Model file for the job. Use its own axes, mm. Face numbers are marked on the shaded views. A direction names the side the tool comes from. Give positions to 0.01 mm unless a question says otherwise; leave off trailing zeros. Loops run counter-clockwise (first coordinate to the right, second up) from the corner with the lowest first, then second, coordinate; pieces in that order, holes last. Notation, with made-up numbers: M -20.5,59 L 4.5,59 A4 ccw 4.5,65 Z; hole C -29.5,-29 d11. An arc over 180 degrees is marked long. Use CSV: the item, a comma, the result in double quotes. Start each with the question number.
(1) Slice it at D-D on x = 5.5. List the corners of the cut face in (y, z), and give its area (3 significant figures).
(2) Slice it at B-B on y = 21.5. List the corners of the cut face in (x, z), and give its area (3 significant figures).
(3) Two-plate mould, pull along Z, no slides. Class the marked faces 6, 7 and 8: pulls with the +Z half, pulls with the -Z half, needs draft (parallel to the pull), parting line crosses it, or undercut.
(4) Tool access for the marked faces 1, 2, 3, 4 and 5: list every direction of +Z, -Z, +X, -X, +Y, -Y with a clear straight run to the whole face (end or side of a thin tool).
(5) Slice it at C-C on z = 0. List the corners of the cut face in (x, y).
(6) Slice it at A-A on x = -3.5. List the corners of the cut face in (y, z).
(7) Flat gauge pins, fed straight in: P1, Ø5, axis at x = -5.5, z = 0, coming from the +Y side; P2, Ø3.5, axis at x = -1, z = 2.5, coming from the +Y side. Where does each tip first touch, or does it go through?
(8) Wall check: line 1 along Z through (x, y) = (10.75, 7.5); line 2 along X through (y, z) = (-0.7, 0); line 3 along Z through (x, y) = (-1, 13). Give the ranges that are in metal, low to high. Write a range as from..to.
```python
from build123d import *

# Parameters (mm, degrees)
SKETCH1_W                = 22
SKETCH1_H                = 11
BOSS_EXTRUDE1_DEPTH      = 23
SKETCH2_W                = 28
SKETCH2_H                = 17
SKETCH2_R                = 3
BOSS_EXTRUDE2_DEPTH      = 2
BOSS_EXTRUDE7_DEPTH      = 28
BOSS_EXTRUDE8_REACH      = 37.025
M5_CLEARANCE_HOLE2_D     = 5.3
M5_CLEARANCE_HOLE2_DEPTH = 2.6


with BuildPart() as part:
    # Sketch1 → Boss-Extrude1 (new body)
    with BuildSketch(Plane(origin=(0, 0, 0), x_dir=(1, 0, 0), z_dir=(0, 1, 0))):
        Polygon((-14, 8.5), (0, 8.5), (14, 8.5), (14, -8.5), (0, -8.5), (-14, -8.5), align=None)
        Rectangle(SKETCH1_W, SKETCH1_H, mode=Mode.SUBTRACT)
    extrude(amount=BOSS_EXTRUDE1_DEPTH)

    # Sketch2 → Boss-Extrude2 (add)
    with BuildSketch(Plane.XZ):
        Rectangle(SKETCH2_W, SKETCH2_H)
        with Locations(Location((-5.5, 0, 0), (0, 0, 270))):
            Circle(SKETCH2_R, mode=Mode.SUBTRACT)
        with Locations(Location((5.5, 0, 0), (0, 0, 270))):
            Circle(SKETCH2_R, mode=Mode.SUBTRACT)
    extrude(amount=BOSS_EXTRUDE2_DEPTH)

    # Sketch10 → Boss-Extrude7 (add, through all)
    with BuildSketch(Plane(origin=(14, 0, 0), x_dir=(0, 0, -1), z_dir=(1, 0, 0))):
        Polygon((16.5, 23), (8.5, 23), (8.5, 9.4), (13.9, 9.4), (13.9, 1), (8.5, 1), (8.5, -2), (16.5, -2), align=None)
    extrude(amount=-BOSS_EXTRUDE7_DEPTH)

    # Sketch11 → Boss-Extrude8 (add, up to next)
    with BuildSketch(Plane.XY.offset(-13.9), mode=Mode.PRIVATE) as boss_extrude8_sk1:
        Polygon((4.575128869, 1), (2.150257739, 5.2), (4.575128869, 9.4), (-4.575128869, 9.4), (-2.150257739, 5.2), (-4.575128869, 1), align=None)
    boss_extrude8_tool1 = extrude(boss_extrude8_sk1.sketch, amount=BOSS_EXTRUDE8_REACH, mode=Mode.PRIVATE) - part.part
    add(boss_extrude8_tool1.solids().sort_by_distance((0, 5.2, -13.9))[0])

    # M5 Clearance Hole2
    with Locations(Plane.XY.offset(-13.9)):
        with Locations((-7, 5.2), (7, 5.2)):
            Hole(M5_CLEARANCE_HOLE2_D / 2, depth=M5_CLEARANCE_HOLE2_DEPTH)


solid = part.part
```
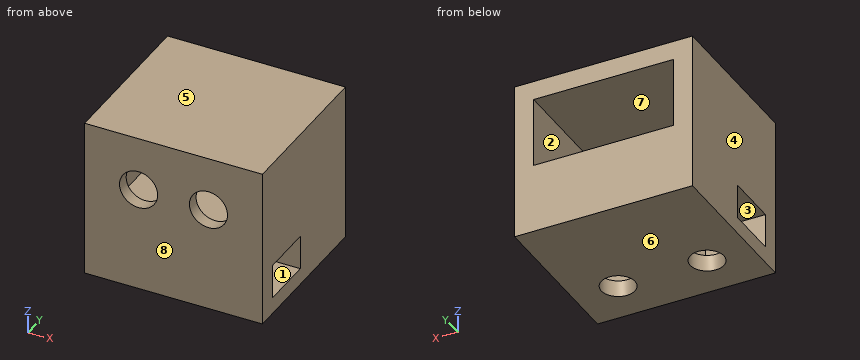
Reply:
1,outline,"M -2,-16.5 L 3.02,-16.5 L 3.02,-13.9 L 1,-13.9 L 1,-8.5 L 9.4,-8.5 L 9.4,-13.9 L 7.38,-13.9 L 7.38,-16.5 L 23,-16.5 L 23,-5.5 L 0,-5.5 L 0,-3 L -2,-3 Z; M -2,3 L 0,3 L 0,5.5 L 23,5.5 L 23,8.5 L -2,8.5 Z"
1,area,"303 mm^2"
2,outline,"M -14,-16.5 L 14,-16.5 L 14,8.5 L -14,8.5 Z; hole M -11,-5.5 L 11,-5.5 L 11,5.5 L -11,5.5 Z"
2,area,"458 mm^2"
3,face 6,"pulls with the -Z half"
3,face 7,"undercut"
3,face 8,"needs draft"
4,face 1,"+X"
4,face 2,"+Y"
4,face 3,"-X"
4,face 4,"+Z, -Z, -X, +Y, -Y"
4,face 5,"+Z, +X, -X, +Y, -Y"
5,outline,"M -14,-2 L -8.5,-2 L -8.5,0 L -11,0 L -11,23 L -14,23 Z; M -2.5,-2 L 2.5,-2 L 2.5,0 L -2.5,0 Z; M 8.5,-2 L 14,-2 L 14,23 L 11,23 L 11,0 L 8.5,0 Z"
6,outline,"M -2,-16.5 L 23,-16.5 L 23,-5.5 L 0,-5.5 L 0,-2.24 L -2,-2.24 Z; M -2,2.24 L 0,2.24 L 0,5.5 L 23,5.5 L 23,8.5 L -2,8.5 Z; hole M 2.86,-13.9 L 7.54,-13.9 L 7.54,-8.5 L 2.86,-8.5 Z"
7,P1,"passes through"
7,P2,"stops at y = 0"
8,line 1,"z = -16.5..-13.9, -8.5..-5.5, 5.5..8.5"
8,line 2,"x = -14..-8.5, -2.5..2.5, 8.5..14"
8,line 3,"z = -16.5..-5.5, 5.5..8.5"
